Could you check a few things on this drawing? It's one solid part, dimensions in mm from its lowest x, y, z. A direction names the side the tool comes from. Give positions to 0.01 mm unless a question says otherwise; leave off trailing zeros. Write each loop counter-clockwise with the first axis right and the second up, starting at its lowest first coordinate (ties: lowest second). Pieces come first, ordered by that corner, then holes. Notation, with made-up numbers: M 17.5,34 L 70.5,34 A16 ccw 70.5,60 Z; hole C 4,-20.75 d4. An arc over 180 degrees is marked long. Write each question's results on one line, items separated by ' | '. Start each with the question number.
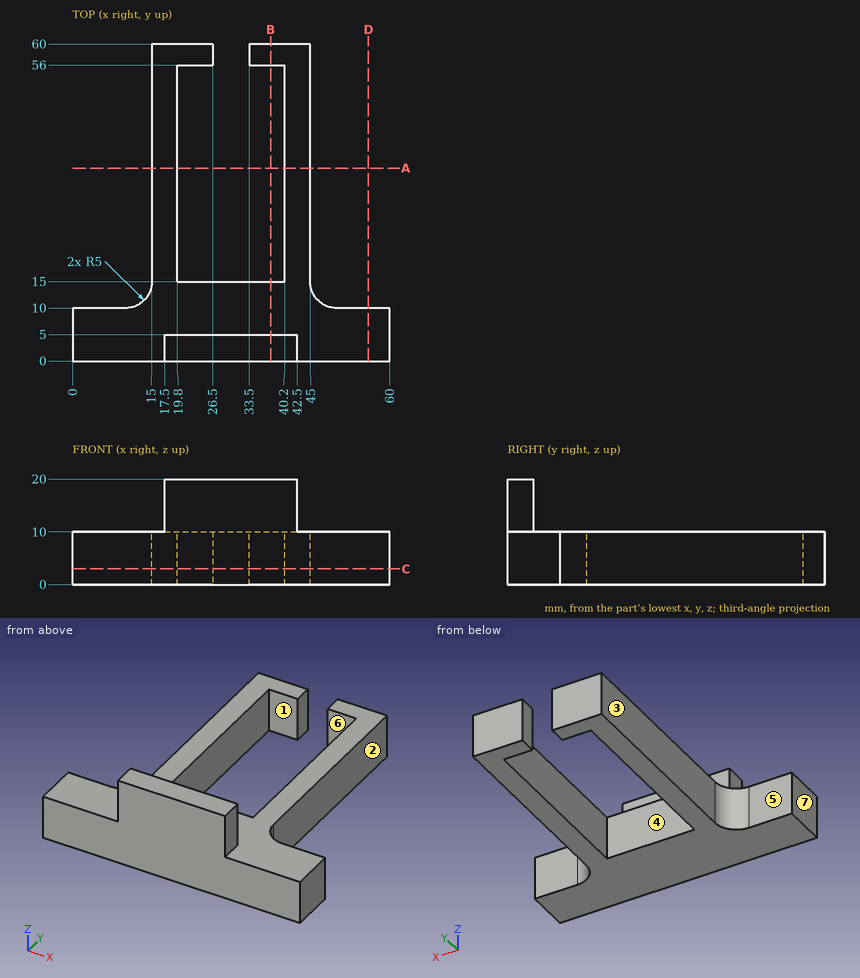
Q1. If we section it at C-C (z = 3): Please give me the cut outline in (x, y), plus the area to 3 significant figures.
Q2. I'm going to push flat-ended pins straight in: P1, Ø2, axis at y = 59, z = 4.5, coming from the -X side; P2, Ø1.5, axis at y = 19, z = 4, coming from the +X side; P3, Ø8, axis at x = 6, z = 11.5, coming from the +Y side; P4, Ø4, axis at x = 29, y = 18, coming from the -Z side. Where does each tip first touch, or does it pass through?
Q3. If we mould it in two halves opening along X, with no side actions, what happens to the marked faces 4, 5, 6 and 7? For each: pulls with the +X half, pulls with the -X half, needs draft (parallel to the pull), parting line crosses it, or undercut.
Q4. For the marked faces 1, 2 and 3, which set-ups out of +Z, -Z, +X, -X, +Y, -Y let a thin tool reach every point of the face, with its end or its side?
Q5. Please list where these lines run through material, in increasing order: line 1 (X direction, y = 33.5, z = 1.25); line 2 (Z direction, x = 55.5, y = 5); line 3 (Y direction, x = 30.5, z = 14). Write a range as [from, to].
Q6. If we section it at D-D (x = 56): Please give me the cut outline in (y, z), plus the area to 3 significant figures.
Q7. If we section it at B-B (x = 37.5): Please give me the cut outline in (y, z).
Q8. If we section it at A-A (y = 36.5): Please give me the cut outline in (x, z), plus the area to 3 significant figures.
Determined:
1) outline: M 0,0 L 60,0 L 60,10 L 50,10 A5 cw 45,15 L 45,60 L 33.5,60 L 33.5,56 L 40.2,56 L 40.2,15 L 19.8,15 L 19.8,56 L 26.5,56 L 26.5,60 L 15,60 L 15,15 A5 cw 10,10 L 0,10 Z | area: 1,250 mm²
2) P1: stops at x = 15 | P2: stops at x = 45 | P3: stops at y = 10 | P4: passes through
3) face 4: undercut | face 5: needs draft | face 6: undercut | face 7: pulls with the -X half
4) face 1: +Z, -Z | face 2: +Z, -Z, +X, +Y | face 3: +Z, -Z, -X, +Y
5) line 1: x = [15, 19.8], [40.2, 45] | line 2: z = [0, 10] | line 3: y = [0, 5]
6) outline: M 0,0 L 10,0 L 10,10 L 0,10 Z | area: 100 mm²
7) outline: M 0,0 L 15,0 L 15,10 L 5,10 L 5,20 L 0,20 Z; M 56,0 L 60,0 L 60,10 L 56,10 Z
8) outline: M 15,0 L 19.8,0 L 19.8,10 L 15,10 Z; M 40.2,0 L 45,0 L 45,10 L 40.2,10 Z | area: 96.0 mm²
